Can you work these out from the model? Positions are in its coordinate system, mm. Face numbers are marked on the shaded views. A direction names the side the tool comes from. Round coordinates to 2 decimals unless told otherwise and drop trailing zeros. Order: outer loops, then holes, each group sorted by start corner. A loop starts at its lowest first (then second) coordinate and runs counter-clockwise, first axis right, second up. Notation, with made-up numbers: (2.5, 72) - (40.5, 72) arc R19 cw to (40.5, 87) - close; hole circle Ø11 at (85, 47.25). An arc over 180 degrees is marked (long way). Write item = value, one per line.
from build123d import *

# Parameters (mm, degrees)
F0_W     = 26.67
F0_H     = 12.7
F1_DEPTH = 12.7
F2_DEPTH = 12.7
F3_SIZE  = 6.35
F4_R     = 0.79375
F5_DEPTH = 25.401
F6_R     = 0.79375
F7_DEPTH = 12.701


with BuildPart() as f1:
    # F0 (on Top) → F1 (new body)
    with BuildSketch(Plane.XY):
        with Locations((32.385, 6.35)):
            Rectangle(F0_W, F0_H)
        with BuildLine():
            ThreePointArc((13.97, 0), (14.639725, 6.486831), (16.620644, 12.7))
            Line((16.620644, 12.7), (0, 12.7))
            Line((0, 12.7), (0, 0))
            Line((0, 0), (13.97, 0))
        make_face()
        Polygon((52.07, 12.7), (45.72, 12.7), (45.72, 0), (45.72, -25.4), (52.07, -25.4), (52.07, 0), align=None)
        with BuildLine():
            Line((19.05, 0), (19.05, 12.7))
            Line((19.05, 12.7), (16.620644, 12.7))
            ThreePointArc((16.620644, 12.7), (14.639725, 6.486831), (13.97, 0))
            Line((13.97, 0), (19.05, 0))
        make_face()
    extrude(amount=F1_DEPTH)

    # F0 (on Top) → F2 (join)
    with BuildSketch(Plane.XY):
        with BuildLine():
            ThreePointArc((13.97, 0), (14.639725, 6.486831), (16.620644, 12.7))
            Line((16.620644, 12.7), (0, 12.7))
            Line((0, 12.7), (0, 0))
            Line((0, 0), (13.97, 0))
        make_face()
        with BuildLine():
            Line((0, 12.7), (16.620644, 12.7))
            ThreePointArc((16.620644, 12.7), (17.7436, 15.012779), (19.05, 17.227118))
            Line((19.05, 17.227118), (19.05, 38.1))
            Line((19.05, 38.1), (0, 38.1))
            Line((0, 38.1), (0, 12.7))
        make_face()
    extrude(amount=-F2_DEPTH)

    # F3
    f3_edges = [f1.edges().sort_by_distance(p)[0] for p in [
        (52.07, 12.7, 6.35),
    ]]
    chamfer(f3_edges, length=F3_SIZE)

    # F4 (on face) → F5 (cut, through all)
    with BuildSketch(Plane.XY.offset(12.7)):
        with Locations((48.895, -6.35)):
            Circle(F4_R)
        with Locations((48.895, -19.05)):
            Circle(F4_R)
    extrude(amount=-F5_DEPTH, mode=Mode.SUBTRACT)

    # F6 (on face) → F7 (cut, through all)
    with BuildSketch(Plane.XY):
        with Locations((9.525, 31.75)):
            Circle(F6_R)
        with Locations((9.712074, 22.225)):
            Circle(F6_R)
    extrude(amount=-F7_DEPTH, mode=Mode.SUBTRACT)


solid = f1.part
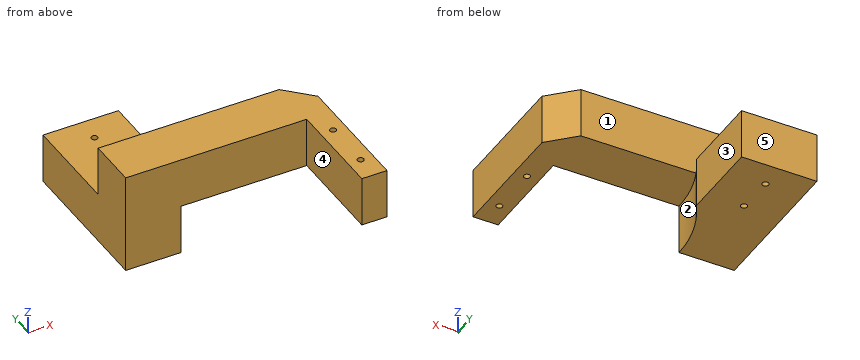
(1) On a 3-axis mill with a long thin cutter (end or side, diameter ignored), from which of +Z, -Z, +X, -X, +Y, -Y can I reach the whole of each face in a straight line? I mean the marked faces 1, 2, 3, 4 and 5. Say none if no direction works.
Computed:
face_1 = +Z, +X, -X, +Y
face_2 = -Z, +X, -Y
face_3 = +Z, -Z, +X, +Y, -Y
face_4 = +Z, -Z, -X, -Y
face_5 = +Z, -Z, +X, -X, +Y
(2) If we section it at A-A (y = 31.75): Write out the boundary of the cut face in (x, z), plus the area to 3 significant figures.
Computed:
outline = (0, -12.7) - (8.73, -12.7) - (8.73, 0) - (0, 0) - close; (10.32, -12.7) - (19.05, -12.7) - (19.05, 0) - (10.32, 0) - close
area = 222 mm^2
(3) Will these pins go through, and if not, where does the flat tip stop? P1, Ø1, axis at x = 48.895, y = -6.35, coming from the +Z side; P2, Ø12, axis at x = 41.5, y = 10.5, coming from the -Z side; P3, Ø6, axis at x = 29.5, z = 6.5, coming from the -Y side; P4, Ø2.5, axis at x = 9.71, y = 22.22, coming from the +Z side.
Computed:
P1 = through
P2 = 0
P3 = 0
P4 = 0
(4) If I drill on line 1 (Y direction, x = 13, z = -9.5); line 2 (Y direction, x = 21, z = 11.75); line 3 (X direction, y = 19.5, z = -11), over which ranges is the centre line in solid material (lowest first)? Write a range as from..to.
Computed:
line_1 = 0..38.1
line_2 = 0..12.7
line_3 = 0..19.05
(5) If we section it at D-D (y = -19.05): Write out the boundary of the cut face in (x, z), plus the area to 3 significant figures.
Computed:
outline = (45.72, 0) - (48.1, 0) - (48.1, 12.7) - (45.72, 12.7) - close; (49.69, 0) - (52.07, 0) - (52.07, 12.7) - (49.69, 12.7) - close
area = 60.5 mm^2
(6) If we section it at B-B (z = 5.5): State how many separate pieces and enclosed holes the cut face has, plus the area to 3 significant figures.
Computed:
separate_pieces = 1
enclosed_holes = 2
area = 798 mm^2
(7) If we section it at C-C (x = 25.5): Write out the boundary of the cut face in (y, z).
Computed:
outline = (0, 0) - (12.7, 0) - (12.7, 12.7) - (0, 12.7) - close
